Input: dimensioned drawing with shaded views. Units: mm. Origin: part minimum x, y, z. A direction names the side the tool comes from. Give positions to 0.01 mm unless a question says otherwise; leave off trailing zeros. Order: outer loops, then holes, each group sorted by start corner. A loop starts at its lowest first (then second) coordinate and runs counter-clockwise, first axis right, second up.
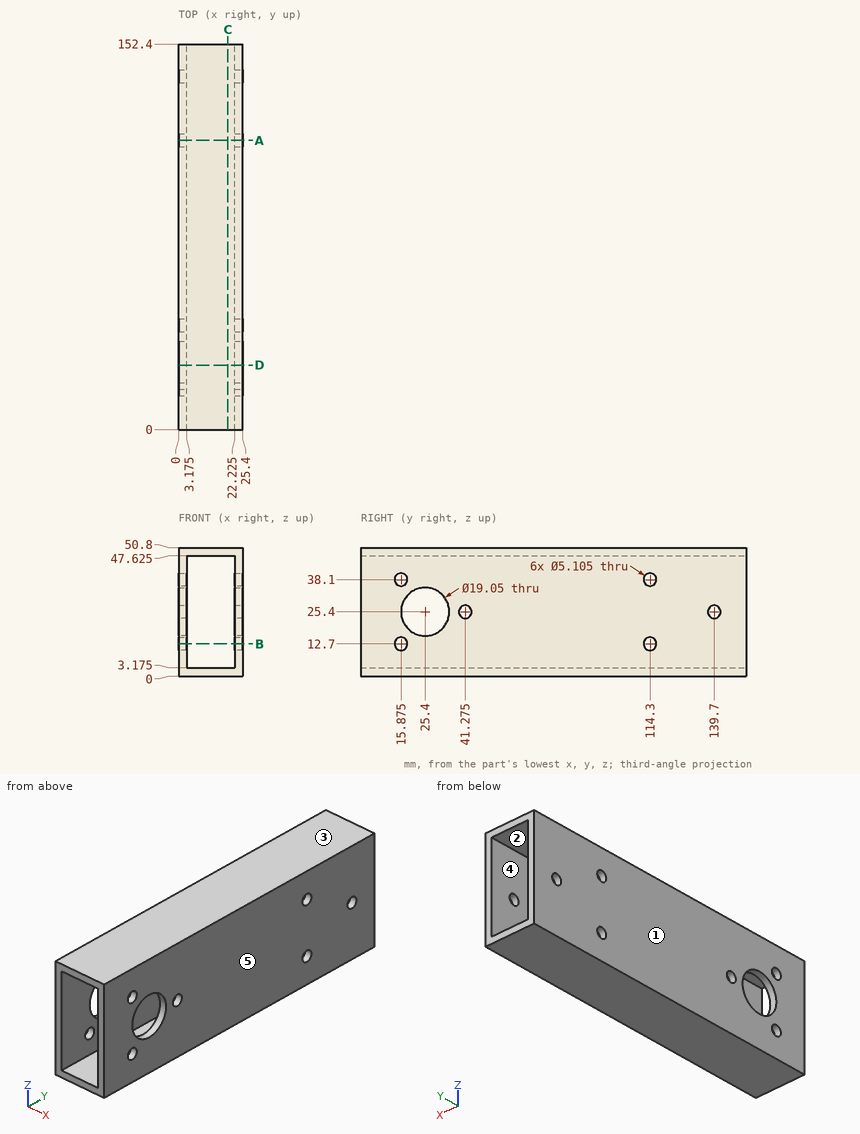
1) Reachability of the marked faces 1 and 2 from +Z, -Z, +X, -X, +Y, -Y: full face, straight path, thin tool, end or side. Return the list, or none.
Report:
face 1: +Z, -Z, -X, +Y, -Y
face 2: +Y, -Y
2) Draft query along X for the marked faces 3, 4 and 5. Return one class per face: +X half, -X half, draft (parallel to the pull), parting line (faces both ways), or undercut.
Report:
face 3: draft
face 4: undercut
face 5: +X half
3) Section query C-C, the plane x = 19.5. Return the cut outline in (y, z) (1 decimal).
Report:
outline: (0, 0) - (152.4, 0) - (152.4, 3.2) - (0, 3.2) - close; (0, 47.6) - (152.4, 47.6) - (152.4, 50.8) - (0, 50.8) - close
4) Pin query (flat end, axial travel): pin 1 (12 mm diameter, centred on x = 21.5, z = 37, fed in from +Y). Return the tip coordinate at first contact, or that it passes through.
Report:
pin 1: stops at y = 152.4
5) Section query D-D, the plane y = 25.4. Return the cut outline in (x, z) (1 decimal).
Report:
outline: (0, 0) - (25.4, 0) - (25.4, 15.9) - (22.2, 15.9) - (22.2, 3.2) - (3.2, 3.2) - (3.2, 15.9) - (0, 15.9) - close; (0, 34.9) - (3.2, 34.9) - (3.2, 47.6) - (22.2, 47.6) - (22.2, 34.9) - (25.4, 34.9) - (25.4, 50.8) - (0, 50.8) - close
6) Section query A-A, the plane y = 114.3. Return the cut outline in (x, z) (1 decimal).
Report:
outline: (0, 0) - (25.4, 0) - (25.4, 10.1) - (22.2, 10.1) - (22.2, 3.2) - (3.2, 3.2) - (3.2, 10.1) - (0, 10.1) - close; (0, 15.3) - (3.2, 15.3) - (3.2, 35.5) - (0, 35.5) - close; (0, 40.7) - (3.2, 40.7) - (3.2, 47.6) - (22.2, 47.6) - (22.2, 40.7) - (25.4, 40.7) - (25.4, 50.8) - (0, 50.8) - close; (22.2, 15.3) - (25.4, 15.3) - (25.4, 35.5) - (22.2, 35.5) - close
7) Section query B-B, the plane z = 12.7. Return the cut outline in (x, y) (1 decimal).
Report:
outline: (0, 0) - (3.2, 0) - (3.2, 13.3) - (0, 13.3) - close; (0, 18.4) - (3.2, 18.4) - (3.2, 111.7) - (0, 111.7) - close; (0, 116.9) - (3.2, 116.9) - (3.2, 152.4) - (0, 152.4) - close; (22.2, 0) - (25.4, 0) - (25.4, 13.3) - (22.2, 13.3) - close; (22.2, 18.4) - (25.4, 18.4) - (25.4, 111.7) - (22.2, 111.7) - close; (22.2, 116.9) - (25.4, 116.9) - (25.4, 152.4) - (22.2, 152.4) - close
8) Material intervals for L1, parallel to Y at x = 1, z = 38.1; L2, parallel to X at y = 32.5, z = 16.5 (1 decimal); L3, parallel to Y at x = 2.25, z = 25.4 (1 decimal), sorted ascending.
Report:
L1: y = 0 to 13.32, 18.43 to 111.75, 116.85 to 152.4
L2: x = 0 to 3.2, 22.2 to 25.4
L3: y = 0 to 15.9, 34.9 to 38.7, 43.8 to 137.1, 142.3 to 152.4
